Geometry check sheet. Reference: drawing and pictorial views, mm from the part's lowest x, y, z. A direction names the side the tool comes from. Round coordinates to 2 decimals unless told otherwise and drop trailing zeros. Order: outer loops, then holes, each group sorted by start corner. A loop starts at its lowest first (then second) coordinate and runs counter-clockwise, first axis right, second up.
(1) Mould release check, pull along Z, two halves, no side actions. Record for the marked faces 4, 5 and 6: released by +Z, released by -Z, zero draft, split by the parting line, or undercut.
(2) Sectioned sample at C-C, the plane z = 46. Enter the section's corners in (x, y) (1 decimal).
(3) Tool access check on the marked faces 1, 2 and 3. Record the directions out of +Z, -Z, +X, -X, +Y, -Y that give a thin tool (end or side, any length) a straight path to the whole face; none if there is none.
(4) Depth check by flat-ended pin: pin 1 (5 mm diameter, centred on y = 5, z = 5.5, fed in from +X); pin 2 (1 mm diameter, centred on x = 29, y = 6.5, fed in from -Z); pin 3 (1.8 mm diameter, centred on x = 44.5, y = 5, fed in from -Z). Enter the tip coordinate at first touch or a pass-through.
(5) Sectioned sample at B-B, the plane x = 44. Enter the section's corners in (y, z) (1 decimal).
(6) Thickness scan on probe 1 along X at (y, z) = (7.25, 24.5); probe 2 along Z at (x, y) = (6, 4.25); probe 3 along Z at (x, y) = (43, 5.75). Record the ranges inside material, lowest first.
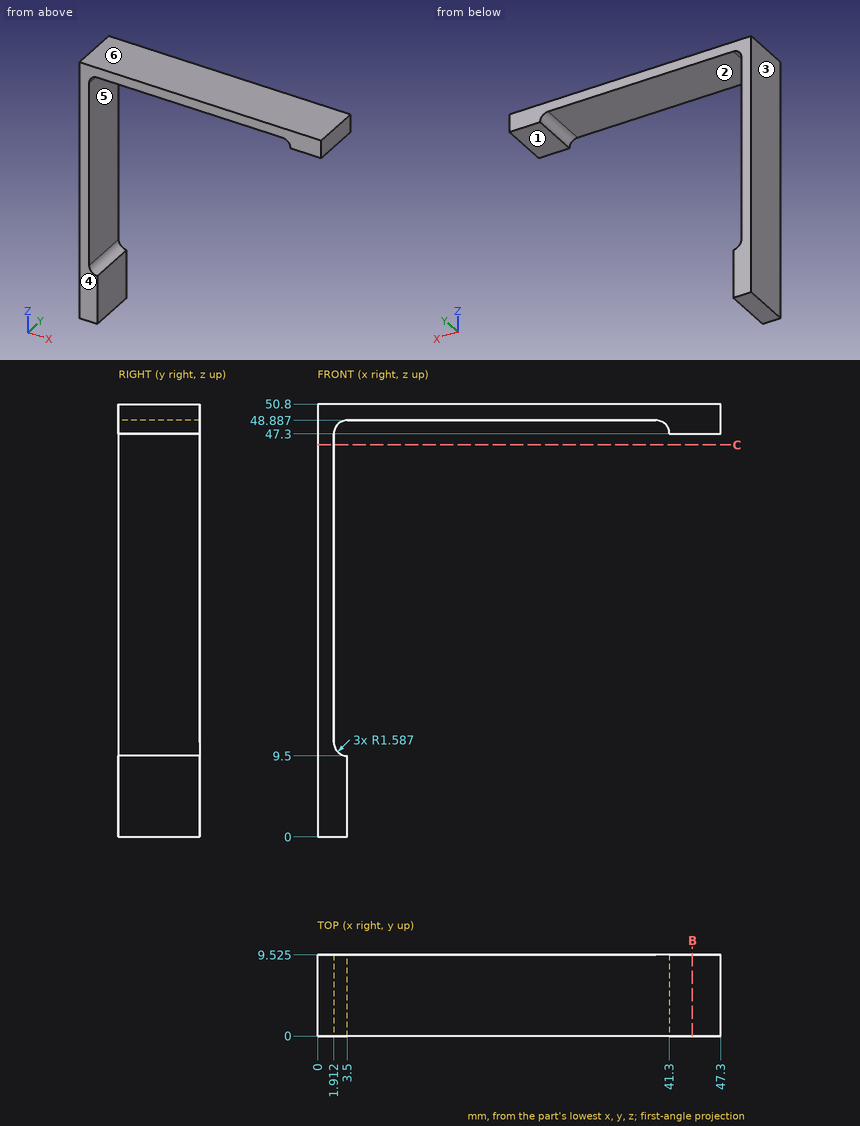
Derived:
1. face 4: zero draft
1. face 5: undercut
1. face 6: released by +Z
2. outline: (0, 0) - (1.9, 0) - (1.9, 9.5) - (0, 9.5) - close
3. face 1: -Z, +X, +Y, -Y
3. face 2: -Z, +Y, -Y
3. face 3: +Z, -Z, -X, +Y, -Y
4. pin 1: stops at x = 3.5
4. pin 2: stops at z = 48.89
4. pin 3: stops at z = 47.3
5. outline: (0, 47.3) - (9.5, 47.3) - (9.5, 50.8) - (0, 50.8) - close
6. probe 1: x = 0 to 1.91
6. probe 2: z = 48.89 to 50.8
6. probe 3: z = 47.3 to 50.8
